Verification items for the finished model (mm, model axes). Round coordinates to 2 decimals unless told otherwise and drop trailing zeros. Loops run counter-clockwise (first coordinate to the right, second up) from the corner with the lowest first, then second, coordinate; pieces in that order, holes last. Notation, with made-up numbers: (37, -13) -> (48, -13) arc R17 cw to (48, 3) -> close; hole circle Ø5 at (-4, 32). An arc over 180 degrees is marked (long way). Use a Markdown table: item, result. Add a question column.
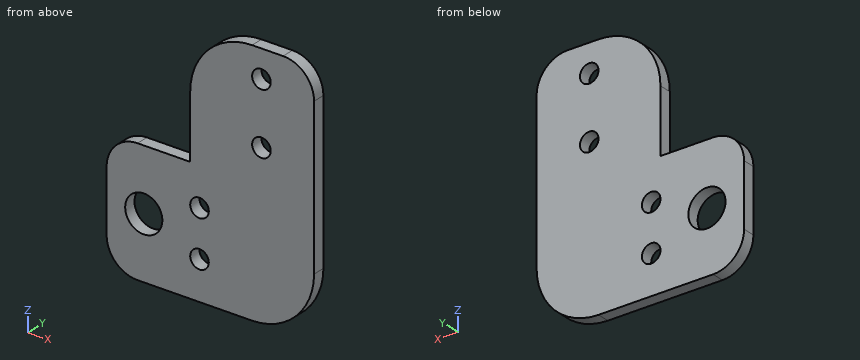
```python
from build123d import *

# Parameters (mm, degrees)
SKETCH1_W           = 25
SKETCH1_H           = 20
BOSS_EXTRUDE1_DEPTH = 2
CUT_EXTRUDE1_REACH  = 18.132
SKETCH2_R           = 1.5
CUT_EXTRUDE2_REACH  = 18.132
SKETCH3_R           = 3
SKETCH4_W           = 20
SKETCH4_H           = 25
BOSS_EXTRUDE2_DEPTH = 2
BOSS_EXTRUDE3_DEPTH = 2
SKETCH6_R           = 1.5
CUT_EXTRUDE3_DEPTH  = 2
SKETCH7_W           = 8.5
SKETCH7_H           = 15.25
BOSS_EXTRUDE5_DEPTH = 2
FILLET1_R           = 10
FILLET2_R           = 5


with BuildPart() as part:
    # Sketch1 → Boss-Extrude1 (new body)
    with BuildSketch(Plane(origin=(0, 0, 0), x_dir=(1, 0, 0), z_dir=(0, 1, 0))):
        Rectangle(SKETCH1_W, SKETCH1_H)
    extrude(amount=BOSS_EXTRUDE1_DEPTH)

    # Sketch2 → Cut-Extrude1 (cut, up to next)
    with BuildSketch(Plane(origin=(0, 2, 0), x_dir=(1, 0, 0), z_dir=(0, 1, 0)), mode=Mode.PRIVATE) as cut_extrude1_sk1:
        with Locations(Location((-6.5, 0, 0), (0, 0, 270))):
            Circle(SKETCH2_R)
    cut_extrude1_tool1 = extrude(cut_extrude1_sk1.sketch, amount=-CUT_EXTRUDE1_REACH, mode=Mode.PRIVATE) & part.part
    # Sketch2 → Cut-Extrude1 (cut, up to next)
    with BuildSketch(Plane(origin=(0, 2, 0), x_dir=(1, 0, 0), z_dir=(0, 1, 0)), mode=Mode.PRIVATE) as cut_extrude1_sk2:
        with Locations(Location((2.5, 3.75, 0), (0, 0, 270))):
            Circle(SKETCH2_R)
    cut_extrude1_tool2 = extrude(cut_extrude1_sk2.sketch, amount=-CUT_EXTRUDE1_REACH, mode=Mode.PRIVATE) & part.part
    # Sketch2 → Cut-Extrude1 (cut, up to next)
    with BuildSketch(Plane(origin=(0, 2, 0), x_dir=(1, 0, 0), z_dir=(0, 1, 0)), mode=Mode.PRIVATE) as cut_extrude1_sk3:
        with Locations(Location((2.5, -3.75, 0), (0, 0, 270))):
            Circle(SKETCH2_R)
    cut_extrude1_tool3 = extrude(cut_extrude1_sk3.sketch, amount=-CUT_EXTRUDE1_REACH, mode=Mode.PRIVATE) & part.part
    add(cut_extrude1_tool1.solids().sort_by_distance((-6.5, 2, 0))[0], mode=Mode.SUBTRACT)
    add(cut_extrude1_tool2.solids().sort_by_distance((2.5, 2, -3.75))[0], mode=Mode.SUBTRACT)
    add(cut_extrude1_tool3.solids().sort_by_distance((2.5, 2, 3.75))[0], mode=Mode.SUBTRACT)

    # Sketch3 → Cut-Extrude2 (cut, up to next)
    with BuildSketch(Plane(origin=(0, 0, 0), x_dir=(-1, 0, 0), z_dir=(0, -1, 0)), mode=Mode.PRIVATE) as cut_extrude2_sk1:
        with Locations(Location((6.5, 0, 0), (0, 0, 90))):
            Circle(SKETCH3_R)
    cut_extrude2_tool1 = extrude(cut_extrude2_sk1.sketch, amount=-CUT_EXTRUDE2_REACH, mode=Mode.PRIVATE) & part.part
    add(cut_extrude2_tool1.solids().sort_by_distance((-6.5, 0, 0))[0], mode=Mode.SUBTRACT)

    # Sketch4 → Boss-Extrude2 (add)
    with BuildSketch(Plane(origin=(0, 2, 0), x_dir=(1, 0, 0), z_dir=(0, 1, 0))):
        with Locations((11, -17.75)):
            Rectangle(SKETCH4_W, SKETCH4_H)
    extrude(amount=-BOSS_EXTRUDE2_DEPTH)

    # Sketch5 → Boss-Extrude3 (add)
    with BuildSketch(Plane(origin=(0, 2, 0), x_dir=(1, 0, 0), z_dir=(0, 1, 0))):
        Polygon((12.5, 10), (12.5, -5.25), (21, -5.25), align=None)
    extrude(amount=-BOSS_EXTRUDE3_DEPTH)

    # Sketch6 → Cut-Extrude3 (cut)
    with BuildSketch(Plane(origin=(0, 2, 0), x_dir=(1, 0, 0), z_dir=(0, 1, 0))):
        with Locations(Location((12.5, -15.75, 0), (0, 0, 270))):
            Circle(SKETCH6_R)
        with Locations(Location((12.5, -25.75, 0), (0, 0, 270))):
            Circle(SKETCH6_R)
    extrude(amount=-CUT_EXTRUDE3_DEPTH, mode=Mode.SUBTRACT)

    # Sketch7 → Boss-Extrude5 (add)
    with BuildSketch(Plane(origin=(0, 2, 0), x_dir=(1, 0, 0), z_dir=(0, 1, 0))):
        with Locations((16.75, 2.375)):
            Rectangle(SKETCH7_W, SKETCH7_H)
    extrude(amount=-BOSS_EXTRUDE5_DEPTH)

    # Fillet1
    fillet1_edges = [part.edges().sort_by_distance(p)[0] for p in [
        (1, 1, 30.25),
        (21, 1, -10),
    ]]
    fillet(fillet1_edges, radius=FILLET1_R)

    # Fillet2
    fillet2_edges = [part.edges().sort_by_distance(p)[0] for p in [
        (21, 1, 30.25),
        (-12.5, 1, 10),
        (-12.5, 1, -10),
    ]]
    fillet(fillet2_edges, radius=FILLET2_R)


solid = part.part
```
1) Thickness scan on line 1 (X direction, y = 0.5, z = 15.75); line 2 (X direction, y = 0.4, z = -2.5); line 3 (X direction, y = 0.4, z = 3.75). Record the ranges inside material, lowest first.
2) Sectioned sample at C-C on x = -6.5. Enter the section's corners in (y, z).
3) Sectioned sample at B-B on y = 1.6. Enter the section's corners in (x, z).
4) Sectioned sample at A-A on z = 3.75. Enter the section's corners in (x, y), then the cut area to 3 significant figures.
5) Sectioned sample at D-D on x = 3.5. Enter the section's corners in (y, z).
6) Go/stop test with flat-tipped pins: pin 1 (12 mm diameter, centred on x = 13, z = 25.5, fed in from -Y); pin 2 (2.5 mm diameter, centred on x = 12.5, z = 15.75, fed in from +Y); pin 3 (1 mm diameter, centred on x = -2, y = 0.5, fed in from +Z). Record where each tip stops, or that it passes through.
Geometry results:
| question | item | result |
|---|---|---|
| 1 | line 1 | 1 to 11, 14 to 21 |
| 1 | line 2 | -12.5 to -8.16, -4.84 to 1.67, 3.33 to 20.68 |
| 1 | line 3 | -12.5 to 1, 4 to 21 |
| 2 | outline | (0, -10) -> (2, -10) -> (2, -3) -> (0, -3) -> close; (0, 3) -> (2, 3) -> (2, 10) -> (0, 10) -> close |
| 3 | outline | (-12.5, -5) arc R5 ccw to (-7.5, -10) -> (11, -10) arc R10 ccw to (21, 0) -> (21, 25.25) arc R5 ccw to (16, 30.25) -> (11, 30.25) arc R10 ccw to (1, 20.25) -> (1, 10) -> (-7.5, 10) arc R5 ccw to (-12.5, 5) -> close; hole circle Ø6 at (-6.5, 0); hole circle Ø3 at (2.5, -3.75); hole circle Ø3 at (2.5, 3.75); hole circle Ø3 at (12.5, 15.75); hole circle Ø3 at (12.5, 25.75) |
| 4 | outline | (-12.5, 0) -> (1, 0) -> (1, 2) -> (-12.5, 2) -> close; (4, 0) -> (21, 0) -> (21, 2) -> (4, 2) -> close |
| 4 | area | 61.0 mm^2 |
| 5 | outline | (0, -10) -> (2, -10) -> (2, -4.87) -> (0, -4.87) -> close; (0, -2.63) -> (2, -2.63) -> (2, 2.63) -> (0, 2.63) -> close; (0, 4.87) -> (2, 4.87) -> (2, 26.86) -> (0, 26.86) -> close |
| 6 | pin 1 | y = 0 |
| 6 | pin 2 | through |
| 6 | pin 3 | z = 10 |
